from build123d import *

# Parameters (mm, degrees)
SKETCH_1_R          = 12.5
EXTRUDE_1_DEPTH     = 55.5
SKETCH_2_R          = 13
EXTRUDE_1_2_DEPTH   = 29
SKETCH_3_R          = 7
EXTRUDE_2_DEPTH     = 2
SKETCH_4_R          = 5
EXTRUDE_3_DEPTH     = 2.5
SKETCH_5_R          = 2.5
EXTRUDE_4_DEPTH     = 12.8
SKETCH_6_R          = 1.5
CUT_EXTRUDE_1_DEPTH = 4


with BuildPart() as part:
    # 스케치1 → Extrude 1 (new body)
    with BuildSketch(Plane.XY):
        Circle(SKETCH_1_R)
    extrude(amount=EXTRUDE_1_DEPTH)

    # 스케치2 → Extrude 1 2 (add)
    with BuildSketch(Plane.XY.offset(55.5)):
        with Locations(Location((0, 0, 0), (0, 0, 180))):
            Circle(SKETCH_2_R)
    extrude(amount=EXTRUDE_1_2_DEPTH)

    # 스케치3 → 보스-돌출2 (add)
    with BuildSketch(Plane.XY.offset(84.5)):
        Circle(SKETCH_3_R)
    extrude(amount=EXTRUDE_2_DEPTH)

    # 스케치4 → 보스-돌출3 (add)
    with BuildSketch(Plane.XY.offset(86.5)):
        Circle(SKETCH_4_R)
    extrude(amount=EXTRUDE_3_DEPTH)

    # 스케치5 → 보스-돌출4 (add)
    with BuildSketch(Plane.XY.offset(89)):
        Circle(SKETCH_5_R)
    extrude(amount=EXTRUDE_4_DEPTH)

    # 스케치6 → 컷-돌출1 (cut)
    with BuildSketch(Plane.XY.offset(84.5)):
        with Locations((0, 10)):
            Circle(SKETCH_6_R)
        with Locations((10, 0)):
            Circle(SKETCH_6_R)
        with Locations((0, -10)):
            Circle(SKETCH_6_R)
        with Locations((-10, 0)):
            Circle(SKETCH_6_R)
    extrude(amount=-CUT_EXTRUDE_1_DEPTH, mode=Mode.SUBTRACT)


solid = part.part
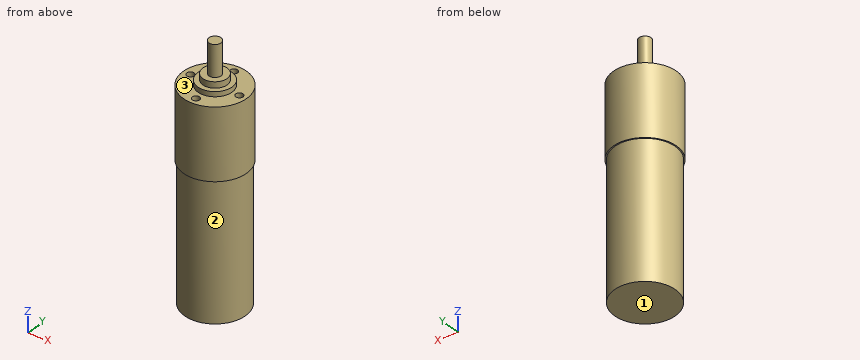
CAD build for the part. Positions are in the model's coordinates, mm. Face numbers are marked on the shaded views. A direction names the side the tool comes from. Give positions to 0.01 mm unless a question says otherwise; leave off trailing zeros. Loops run counter-clockwise (first coordinate to the right, second up) from the corner with the lowest first, then second, coordinate; pieces in that order, holes last. Notation, with made-up numbers: M 20,-26.5 L 55,-26.5 A20 cw 55,-6.5 Z; hole C 86,-17 d5. An arc over 180 degrees is marked long. Answer in a Markdown table with one row per item. Add a question column.
Item 1: Band-saw the part on C-C on z = 77. Give the cut face in (x, y).
Item 2: Tool access for the marked faces 1, 2 and 3: list every direction of +Z, -Z, +X, -X, +Y, -Y with a clear straight run to the whole face (end or side of a thin tool).
Item 3: Probe probe 1 along Y at (x, z) = (0, 83.2); probe 2 along Z at (x, y) = (3.5, -8); probe 3 along Z at (x, y) = (-3.75, -1.75). List the from-to ranges inside material, lowest first.
Item 4: Band-saw the part on D-D on y = -4. Give the cut face in (x, z), then the cut area to 3 significant figures.
Item 5: Drop flat-ended pins along their axis: P1, Ø12, axis at x = -8, z = 26.5, coming from the -Y side; P2, Ø3.5, axis at x = 0, y = -10, coming from the +Z side; P3, Ø5, axis at y = 3, z = 88.5, coming from the -X side. Give the stop position or say it passes through.
Item 6: Band-saw the part on A-A on x = 0. Give the cut face in (y, z).
Reply:
| question | item | result |
|---|---|---|
| 1 | outline | C 0,0 d26 |
| 2 | face 1 | -Z, +X, -X, +Y, -Y |
| 2 | face 2 | -Z |
| 2 | face 3 | +Z |
| 3 | probe 1 | y = -13 to -11.5, -8.5 to 8.5, 11.5 to 13 |
| 3 | probe 2 | z = 0 to 84.5 |
| 3 | probe 3 | z = 0 to 89 |
| 4 | outline | M -12.37,55.5 L -11.84,55.5 L -11.84,0 L 11.84,0 L 11.84,55.5 L 12.37,55.5 L 12.37,84.5 L 5.74,84.5 L 5.74,86.5 L 3,86.5 L 3,89 L -3,89 L -3,86.5 L -5.74,86.5 L -5.74,84.5 L -12.37,84.5 Z |
| 4 | area | 2,070 mm^2 |
| 5 | P1 | stops at y = -12.34 |
| 5 | P2 | stops at z = 84.5 |
| 5 | P3 | stops at x = -6.84 |
| 6 | outline | M -13,55.5 L -12.5,55.5 L -12.5,0 L 12.5,0 L 12.5,55.5 L 13,55.5 L 13,84.5 L 11.5,84.5 L 11.5,80.5 L 8.5,80.5 L 8.5,84.5 L 7,84.5 L 7,86.5 L 5,86.5 L 5,89 L 2.5,89 L 2.5,101.8 L -2.5,101.8 L -2.5,89 L -5,89 L -5,86.5 L -7,86.5 L -7,84.5 L -8.5,84.5 L -8.5,80.5 L -11.5,80.5 L -11.5,84.5 L -13,84.5 Z |
